The model under review builds one solid part; all positions refer to its coordinate system, in mm. A direction names the side the tool comes from. Coordinates: 2 decimals unless noted, no trailing zeros. Loops run counter-clockwise (first coordinate to the right, second up) from the corner with the lowest first, then second, coordinate; pieces in that order, holes last. Notation, with made-up numbers: (-27, 7) - (15, 7) arc R35 ccw to (15, 43) - close; hole circle Ø6 at (-21.5, 81). An arc over 180 degrees is marked (long way). Use a Markdown table: item, result. Add a question column.
1) To check wall thickness, follow L1, parallel to Z at x = 0, y = 5.5; L2, parallel to Y at x = -0.25, z = 0.65. State the ranges of each line that lie inside material, in increasing order. Write a range as [from, to].
2) The part is to be moulded in two halves that separate along Z. For faces 1 (the flat face through (-1.2, 7, 1.1)), 2 (the flat face through (0, 1, 0)), 3 (the flat face through (1, 10, -1)), say which applies: pulls with the +Z half, pulls with the -Z half, needs draft (parallel to the pull), parting line crosses it, or undercut.
3) For faces 4 (the flat face through (-1.2, 7, -1.2)), 5 (the cylindrical face through (0, 5, -2)), 6 (the flat face through (1.1, 7, -1.2)), 7 (the flat face through (1.14, 7, 1.14)), 8 (the flat face through (0, 0.5, 0.4)), list the 3-axis set-ups (+Z, -Z, +X, -X, +Y, -Y) from which the entire face can be reached by the end or side of a thin tool; tool diameter is ignored.
4) Add section B-B, the plane y = 6.5. Give the boundary of the cut face in (x, z).
5) Add section A-A, the plane y = 11.75. Give the boundary of the cut face in (x, z), and give its area (3 significant figures).
6) Clearance check with flat-ended pins moving along their axes: pin 1 (0.5 mm diameter, centred on x = -1.5, y = 0.5, fed in from +Z); pin 2 (3 mm diameter, centred on x = 0.5, y = 9.5, fed in from +Z). State where each tip first meets the part, or that it passes through.
Autodesk Inventor part; units mm, degrees
ref_plane "YZ Plane" through (0, 0, 0) normal (1, 0, 0) x (0, 1, 0)
ref_plane "XZ Plane" through (0, 0, 0) normal (0, 1, 0) x (-1, 0, 0)
ref_plane "XY Plane" through (0, 0, 0) normal (0, 0, 1) x (1, 0, 0)
sketch "Sketch1" plane through (0, 0, 0) normal (0, 1, 0) x (-1, 0, 0)
  circle A0 centre (0, 0) radius 2.9
  dimension "d0" = 5.8
extrude "Extrusion1" add sketch "Sketch1" along normal blind 3
sketch "Sketch2" plane through (0, 3, 0) normal (0, 1, 0) x (1, 0, 0)
  circle A0 centre (0, 0) radius 2
  dimension "d3" = 4
extrude "Extrusion2" add sketch "Sketch2" along normal blind 4
sketch "Sketch3" plane through (0, 7, 0) normal (0, 1, 0) x (1, 0, 0)
  circle A0 centre (0, 0) radius 2
  line L0 (0, -2) -> (-2, 0)
  line L1 (-2, 0) -> (0, 2)
  line L2 (0, 2) -> (2, 0)
  line L3 (2, 0) -> (0, -2)
extrude "Extrusion3" add sketch "Sketch3" along normal blind 5.5 contours L3 L0 L1 L2
fillet "Fillet1" radius 1 1 edges at (2.9, 3, 0)
fillet "Fillet2" radius 0.5 1 edges at (2.9, 0, 0)
sketch "Sketch4" plane through (0, 0, 0) normal (0, -1, 0) x (1, 0, 0)
  line L0 (0, 0) -> (-2.9, 0)
  circle A0 centre (0, 0) radius 2.9
  line L1 (0, 0) -> (2.973, 0)
  line L2 (-2.9, 0.4) -> (0, 0.4)
  line L3 (0, 0.4) -> (2.973, 0.4)
  line L4 (-2.9, -0.4) -> (0, -0.4)
  line L5 (0, -0.4) -> (2.973, -0.4)
  circle A1 centre (0, 0) radius 2.9275
  point P0 (2.8723, -0.4)
  point P1 (2.8723, 0.4)
  point P2 (-2.8723, 0.4)
  point P3 (-2.8723, -0.4)
  dimension "d10" = 0.4
  dimension "d11" = 0.4
extrude "Extrusion4" cut sketch "Sketch4" against normal blind 1 contours L1 A0 L5 L4 L0 | L0 A0 L2 L3 L1
sketch "Sketch5" plane through (0, 12.5, 0) normal (0, 1, 0) x (1, 0, 0)
  circle A0 centre (0, 0) radius 1
  dimension "d14" = 2
extrude "Extrusion5" cut sketch "Sketch5" against normal blind 11
properties part number "sroub"
From the geometry:
| question | item | result |
|---|---|---|
| 1 | L1 | z = [-2, -1], [1, 2] |
| 1 | L2 | y = [0, 1.5] |
| 2 | face 1 | needs draft |
| 2 | face 2 | undercut |
| 2 | face 3 | pulls with the -Z half |
| 3 | face 4 | -Z, -X, +Y |
| 3 | face 5 | +Y |
| 3 | face 6 | -Z, +X, +Y |
| 3 | face 7 | +Z, +X, +Y |
| 3 | face 8 | +X, -X, -Y |
| 4 | outline | circle Ø4 at (0, 0); hole circle Ø2 at (0, 0) |
| 5 | outline | (-2, 0) - (0, -2) - (2, 0) - (0, 2) - close; hole circle Ø2 at (0, 0) |
| 5 | area | 4.86 mm^2 |
| 6 | pin 1 | stops at z = 2.62 |
| 6 | pin 2 | stops at z = 2 |
